from build123d import *

# Parameters (mm, degrees)
EXTRUDE_1_DEPTH     = 1
SKETCH_6_W          = 6.979999977
SKETCH_6_H          = 23.78
CUT_EXTRUDE_1_DEPTH = 0.5
FILLET_1_R          = 0.7


with BuildPart() as part:
    # 草图1 → 凸台-拉伸1 (new body)
    with BuildSketch(Plane.XY):
        with BuildLine():
            Line((-5.268787068, -23.395653078), (-5.268787078, -52.29634699))
            add(Edge.make_bspline(
                [(-5.268787078, -52.29634699), (-5.268787078, -52.990318083), (-5.137001379, -54.080149918), (-4.182317261, -55.003717165), (-3.39928825, -55.373199943), (-2.383654985, -55.567305407), (-1.243870186, -55.650276692), (-0.457601939, -55.692931511), (-0.012274069, -55.692882673)],
                knots=[0, 0, 0, 0, 0.301160008, 0.404454001, 0.537204471, 0.652206641, 0.831341381, 1, 1, 1, 1], degree=3))
            add(Edge.make_bspline(
                [(-0.012274069, -55.692882673), (0.433053802, -55.692931511), (1.219322049, -55.650276693), (2.359106848, -55.567305408), (3.374740114, -55.373199945), (4.157769124, -55.003717168), (5.112453243, -54.080149921), (5.244238943, -52.990318087), (5.244238943, -52.296346994)],
                knots=[0, 0, 0, 0, 0.168658619, 0.347793359, 0.462795529, 0.595545999, 0.698839992, 1, 1, 1, 1], degree=3))
            Line((5.244238943, -52.296346994), (5.244238953, -23.395653081))
            add(Edge.make_bspline(
                [(5.244238953, -23.395653081), (5.244238953, -22.701681988), (5.112453254, -21.611850154), (4.157769136, -20.688282907), (3.374740126, -20.318800129), (2.359106861, -20.124694665), (1.219322061, -20.041723379), (0.433053814, -19.999068561), (-0.012274056, -19.999117399)],
                knots=[0, 0, 0, 0, 0.301160008, 0.404454001, 0.537204471, 0.652206641, 0.831341381, 1, 1, 1, 1], degree=3))
            add(Edge.make_bspline(
                [(-0.012274056, -19.999117399), (-0.457601926, -19.999068561), (-1.243870174, -20.041723378), (-2.383654973, -20.124694663), (-3.399288238, -20.318800126), (-4.182317249, -20.688282904), (-5.137001368, -21.61185015), (-5.268787067, -22.701681985), (-5.268787068, -23.395653078)],
                knots=[0, 0, 0, 0, 0.168658619, 0.347793359, 0.462795529, 0.595545999, 0.698839992, 1, 1, 1, 1], degree=3))
        make_face()
    extrude(amount=EXTRUDE_1_DEPTH)

    # 草图6 → 切除-拉伸1 (cut)
    with BuildSketch(Plane.XY.offset(1)):
        with Locations((-0.012274056, -40.222000037)):
            Rectangle(SKETCH_6_W, SKETCH_6_H)
    extrude(amount=-CUT_EXTRUDE_1_DEPTH, mode=Mode.SUBTRACT)

    # 圆角1
    fillet_1_edges = [part.edges().sort_by_distance(p)[0] for p in [
        (3.477725932, -52.112000037, 0.75),
        (-3.502274045, -52.112000037, 0.75),
        (-3.502274045, -28.332000037, 0.75),
        (3.477725932, -28.332000037, 0.75),
    ]]
    fillet(fillet_1_edges, radius=FILLET_1_R)


solid = part.part
Could you check a few things on this model? Use its own coordinates, in mm. Coordinates: 2 decimals unless noted, no trailing zeros. Order: outer loops, then holes, each group sorted by start corner. A loop starts at its lowest first (then second) coordinate and runs counter-clockwise, first axis right, second up. Notation, with made-up numbers: (38, 16.5) - (95, 16.5) arc R35 ccw to (95, 48.5) - close; hole circle Ø11 at (55, -24). An arc over 180 degrees is marked (long way). Answer in a Markdown table with one row per item. Add a question column.
(1) I need wall thicknesses on L1, parallel to Y at x = 0, z = 0.95; L2, parallel to X at y = -38.5, z = 0.8; L3, parallel to Z at x = -1.25, y = -52. Which ranges of each line are inside material? Lowest first, please.
(2) Will this pin go through, and if not, where does the flat tip stop? pin 1 (3.5 mm diameter, centred on x = -1.5, y = -36, fed in from +Z).
(3) If we mould it in two halves opening along Y, with no side actions, what happens to faces 1 (the face through (-4, -38, 1)), 2 (the face through (0, -40, 0.5))? For each: released by +Y, released by -Y, zero draft, split by the parting line, or undercut.
(4) If we section it at A-A, the plane y = -30: Please give me the cut outline in (x, z), then the cut area to 3 significant figures.
Results are:
| question | item | result |
|---|---|---|
| 1 | L1 | y = -55.69 to -52.11, -28.33 to -20 |
| 1 | L2 | x = -5.27 to -3.5, 3.48 to 5.24 |
| 1 | L3 | z = 0 to 0.5 |
| 2 | pin 1 | stops at z = 0.5 |
| 3 | face 1 | zero draft |
| 3 | face 2 | undercut |
| 4 | outline | (-5.27, 0) - (5.24, 0) - (5.24, 1) - (3.48, 1) - (3.48, 0.5) - (-3.5, 0.5) - (-3.5, 1) - (-5.27, 1) - close |
| 4 | area | 7.02 mm2 |
